Can you work these out from the drawing? Everything is in mm from the part's minimum corner. A direction names the side the tool comes from. Round coordinates to 2 decimals unless told otherwise and drop trailing zeros. Write each loop counter-clockwise with the first axis right and the second up, starting at its lowest first coordinate (ties: lowest second). Pieces come first, ordered by that corner, then holes. Notation, with made-up numbers: M -9.5,-22.75 L 9.5,-22.75 A8 cw 9.5,-15.75 Z; hole C 28,-16 d3. An arc over 180 degrees is marked long. Answer in a Markdown table with one row per item. Add a question column.
(1) I'm going to push flat-ended pins straight in: pin 1 (10 mm diameter, centred on x = 47.5, y = 38, fed in from -Z); pin 2 (12 mm diameter, centred on x = 54.5, y = 12.5, fed in from +Z); pin 3 (8 mm diameter, centred on x = 78.5, y = 45, fed in from +Z); pin 4 (12.5 mm diameter, centred on y = 67.5, z = 38, fed in from +X). Where does each tip first touch, or does it pass through?
(2) Suppose I cut it at B-B, the plane z = 34. Write out the boundary of the cut face in (x, y).
(3) For the marked faces 1, 2 and 3, which set-ups out of +Z, -Z, +X, -X, +Y, -Y let a thin tool reach every point of the face, with its end or its side?
(4) Suppose I cut it at A-A, the plane y = 48. Write out the boundary of the cut face in (x, z), then the cut area to 3 significant figures.
(5) Suppose I cut it at C-C, the plane x = 75.5. Write out the boundary of the cut face in (y, z), then the cut area to 3 significant figures.
(6) If I drill on probe 1 along X at (y, z) = (61, 31.5); probe 2 along Y at (x, z) = (88, 30); probe 3 along Z at (x, y) = (117, 13), over which ranges is the centre line in solid material (lowest first)?
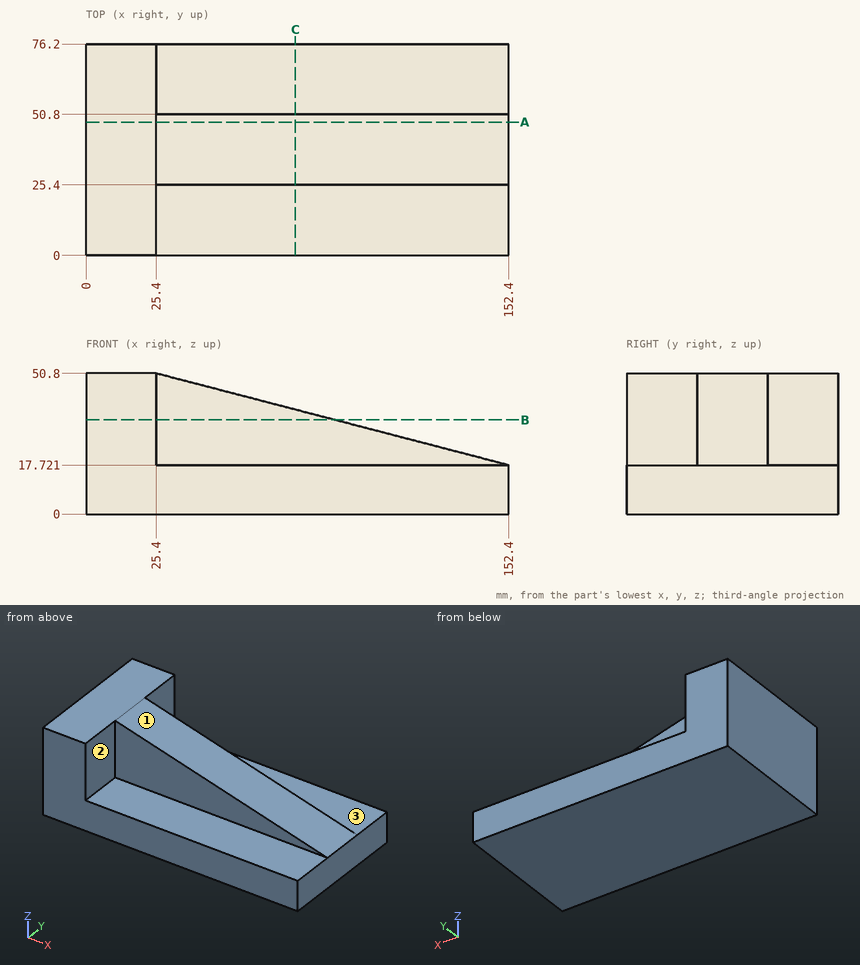
Calculated:
| question | item | result |
|---|---|---|
| 1 | pin 1 | z = 0 |
| 1 | pin 2 | z = 17.72 |
| 1 | pin 3 | z = 38.01 |
| 1 | pin 4 | x = 25.4 |
| 2 | outline | M 0,0 L 25.4,0 L 25.4,25.4 L 89.9,25.4 L 89.9,50.8 L 25.4,50.8 L 25.4,76.2 L 0,76.2 Z |
| 3 | face 1 | +Z, +X, +Y, -Y |
| 3 | face 2 | +Z, +X, -Y |
| 3 | face 3 | +Z, +X, +Y |
| 4 | outline | M 0,0 L 152.4,0 L 152.4,17.72 L 25.4,50.8 L 0,50.8 Z |
| 4 | area | 5,640 mm² |
| 5 | outline | M 0,0 L 76.2,0 L 76.2,17.72 L 50.8,17.72 L 50.8,37.75 L 25.4,37.75 L 25.4,17.72 L 0,17.72 Z |
| 5 | area | 1,860 mm² |
| 6 | probe 1 | 0 to 25.4 |
| 6 | probe 2 | 25.4 to 50.8 |
| 6 | probe 3 | 0 to 17.72 |
